from build123d import *

# Parameters (mm, degrees)
F0_R     = 10
F1_DEPTH = 40
F2_DEPTH = 25


with BuildPart() as f1:
    # F0 (on Top) → F1 (new body)
    with BuildSketch(Plane.XY):
        with BuildLine():
            ThreePointArc((5.697674, 34.533122), (26.68725, 22.644882), (35, 0))
            ThreePointArc((35, 0), (26.68725, -22.644882), (5.697674, -34.533122))
            Line((5.697674, -34.533122), (110.348837, -17.266561))
            ThreePointArc((110.348837, -17.266561), (90, 0), (110.348837, 17.266561))
            Line((110.348837, 17.266561), (5.697674, 34.533122))
        make_face()
        with BuildLine():
            ThreePointArc((125, 0), (120.843625, 11.322441), (110.348837, 17.266561))
            ThreePointArc((110.348837, 17.266561), (90, 0), (110.348837, -17.266561))
            ThreePointArc((110.348837, -17.266561), (120.843625, -11.322441), (125, 0))
        make_face()
        with Locations((107.5, 0)):
            Circle(F0_R, mode=Mode.SUBTRACT)
        with BuildLine():
            ThreePointArc((5.697674, -34.533122), (26.68725, -22.644882), (35, 0))
            ThreePointArc((35, 0), (26.68725, 22.644882), (5.697674, 34.533122))
            ThreePointArc((5.697674, 34.533122), (0, 35), (-5.697674, 34.533122))
            ThreePointArc((-5.697674, 34.533122), (-35, 0), (-5.697674, -34.533122))
            ThreePointArc((-5.697674, -34.533122), (0, -35), (5.697674, -34.533122))
        make_face()
        with BuildLine():
            ThreePointArc((-16.77051, 5), (0, 17.5), (16.77051, 5))
            Line((16.77051, 5), (22.5, 5))
            Line((22.5, 5), (22.5, -5))
            Line((22.5, -5), (16.77051, -5))
            ThreePointArc((16.77051, -5), (0, -17.5), (-16.77051, -5))
            Line((-16.77051, -5), (-22.5, -5))
            Line((-22.5, -5), (-22.5, 5))
            Line((-22.5, 5), (-16.77051, 5))
        make_face(mode=Mode.SUBTRACT)
    extrude(amount=F1_DEPTH)

    # F0 (on Top) → F2 (join)
    with BuildSketch(Plane.XY):
        with BuildLine():
            ThreePointArc((-5.697674, -34.533122), (-35, 0), (-5.697674, 34.533122))
            Line((-5.697674, 34.533122), (-110.348837, 17.266561))
            ThreePointArc((-110.348837, 17.266561), (-96.177559, 13.343625), (-90, 0))
            ThreePointArc((-90, 0), (-96.177559, -13.343625), (-110.348837, -17.266561))
            Line((-110.348837, -17.266561), (-5.697674, -34.533122))
        make_face()
        with BuildLine():
            ThreePointArc((-90, 0), (-96.177559, 13.343625), (-110.348837, 17.266561))
            ThreePointArc((-110.348837, 17.266561), (-125, 0), (-110.348837, -17.266561))
            ThreePointArc((-110.348837, -17.266561), (-96.177559, -13.343625), (-90, 0))
        make_face()
        with Locations((-107.5, 0)):
            Circle(F0_R, mode=Mode.SUBTRACT)
    extrude(amount=F2_DEPTH)


solid = f1.part
Part model, mm, in its own coordinate system. A direction names the side the tool comes from. Coordinates: 2 decimals unless noted, no trailing zeros. Loops run counter-clockwise (first coordinate to the right, second up) from the corner with the lowest first, then second, coordinate; pieces in that order, holes last. Notation, with made-up numbers: (52, 2.25) - (88, 2.25) arc R21 cw to (88, 14.25) - close; hole circle Ø2 at (33, -21). An arc over 180 degrees is marked (long way). Write each question's results on one line, items separated by ' | '. Start each with the question number.
Q1. Which spindle directions (+Z, -Z, +X, -X, +Y, -Y) get a long thin tool onto all of the face, cutting with end or side? Do faces 1 (the flat face through (20, 5, 20)), 2 (the flat face through (-58.76, -25.78, 12.32)). Say none if no direction does.
Q2. Two-plate mould, pull along Y, no slides. Class faces 3 (the flat face through (20, -5, 20)), 4 (the flat face through (-20, -5, 20)), 5 (the cylindrical face through (-125, 0, 12)), 6 (the flat face through (-2, -23, 0)): +Y half, -Y half, draft (parallel to the pull), parting line (faces both ways), or undercut.
Q3. Probe line 1 along X through (y, z) = (-7, 19.5); line 2 along Y through (x, z) = (-107, 19); line 3 along Y through (x, z) = (-17, 17). List the from-to ranges inside material, lowest first.
Q4. Slice it at D-D on z = 19.5. Give the cut face in (x, y), and give its area (3 significant figures).
Q5. Drop flat-ended pins along their axis: pin 1 Ø6.5 at (x, z) = (-18.5, 15) entering from +Y; pin 2 Ø6 at (x, z) = (70, 15.5) entering from -Y; pin 3 Ø6.5 at (x, z) = (-20, 17) entering from -Y. Give the stop position or say it passes through.
Q6. Slice it at B-B on x = 107.5. Give the cut face in (y, z).
Q7. Slice it at A-A on z = 32. Give the cut face in (x, y).
Q8. Slice it at C-C on y = 7.5. Give the cut face in (x, z).
Answer:
1) face 1: +Z, -Z | face 2: +Z, -Z, -X, -Y
2) face 3: undercut | face 4: undercut | face 5: parting line | face 6: draft
3) line 1: x = -123.54 to -114.64, -100.36 to -16.04, 16.04 to 100.36, 114.64 to 123.54 | line 2: y = -17.82 to -9.99, 9.99 to 17.82 | line 3: y = -32.67 to -5, 5 to 32.67
4) outline: (-110.35, -17.27) - (-5.7, -34.53) arc R35 ccw to (5.7, -34.53) - (110.35, -17.27) arc R17.5 ccw to (110.35, 17.27) - (5.7, 34.53) arc R35 ccw to (-5.7, 34.53) - (-110.35, 17.27) arc R17.5 ccw to start; hole circle Ø20 at (-107.5, 0); hole (-22.5, -5) - (-16.77, -5) arc R17.5 ccw to (16.77, -5) - (22.5, -5) - (22.5, 5) - (16.77, 5) arc R17.5 ccw to (-16.77, 5) - (-22.5, 5) - close; hole circle Ø20 at (107.5, 0) | area: 10,700 mm2
5) pin 1: stops at y = 32.96 | pin 2: stops at y = -24.42 | pin 3: stops at y = -32.71
6) outline: (-17.74, 0) - (-10, 0) - (-10, 40) - (-17.74, 40) - close; (10, 0) - (17.74, 0) - (17.74, 40) - (10, 40) - close
7) outline: (-5.7, -34.53) arc R35 ccw to (5.7, -34.53) - (110.35, -17.27) arc R17.5 ccw to (110.35, 17.27) - (5.7, 34.53) arc R35 ccw to (-5.7, 34.53) arc R35 ccw to start; hole (-22.5, -5) - (-16.77, -5) arc R17.5 ccw to (16.77, -5) - (22.5, -5) - (22.5, 5) - (16.77, 5) arc R17.5 ccw to (-16.77, 5) - (-22.5, 5) - close; hole circle Ø20 at (107.5, 0)
8) outline: (-123.31, 0) - (-114.11, 0) - (-114.11, 25) - (-123.31, 25) - close; (-100.89, 0) - (-15.81, 0) - (-15.81, 40) - (-34.19, 40) - (-34.19, 25) - (-100.89, 25) - close; (15.81, 0) - (100.89, 0) - (100.89, 40) - (15.81, 40) - close; (114.11, 0) - (123.31, 0) - (123.31, 40) - (114.11, 40) - close
